```python
from build123d import *

# Parameters (mm, degrees)
SKETCH1_R                = 2
EXTRUDE1_DEPTH           = 3.125
ESBO_O1_R                = 12
ESBO_O1_R_2              = 2
RESSALTO_EXTRUS_O1_DEPTH = 1
FILETE1_R                = 1


with BuildPart() as part:
    # Sketch1 → Extrude1 (new body)
    with BuildSketch(Plane(origin=(0, 0, 0), x_dir=(1, 0, 0), z_dir=(0, 1, 0))):
        Polygon((3.859462612, 2.263930582), (-0.030890091, 4.474357958), (-3.890352703, 2.210427376), (-3.859462612, -2.263930582), (0.030890091, -4.474357958), (3.890352703, -2.210427376), align=None)
        with Locations(Location((0, 0, 0), (0, 0, 270))):  # turned: the seam where the file's is
            Circle(SKETCH1_R, mode=Mode.SUBTRACT)
    extrude(amount=EXTRUDE1_DEPTH)

    # Esboço1 → Ressalto-extrusão1 (add)
    with BuildSketch(Plane(origin=(0, 3.125, 0), x_dir=(1, 0, 0), z_dir=(0, 1, 0))):
        with Locations(Location((0, 0, 0), (0, 0, 270))):  # turned: the seam where the file's is
            Circle(ESBO_O1_R)
        with Locations(Location((0, 0, 0), (0, 0, 270))):  # turned: the seam where the file's is
            Circle(ESBO_O1_R_2, mode=Mode.SUBTRACT)
    extrude(amount=RESSALTO_EXTRUS_O1_DEPTH)

    # Filete1
    filete1_edges = [part.edges().sort_by_distance(p)[0] for p in [
        (-1.960621397, 3.125, -3.342392667),
        (-3.874907657, 3.125, 0.026751603),
        (-1.91428626, 3.125, 3.36914427),
        (1.960621397, 3.125, 3.342392667),
        (3.874907657, 3.125, -0.026751603),
        (1.91428626, 3.125, -3.36914427),
    ]]
    fillet(filete1_edges, radius=FILETE1_R)


solid = part.part
```
Source: CAD feature listing. Evaluate the final solid. Frame: model axes, mm. A direction names the side the tool comes from. Round coordinates to 2 decimals unless told otherwise and drop trailing zeros. Loops run counter-clockwise (first coordinate to the right, second up) from the corner with the lowest first, then second, coordinate; pieces in that order, holes last.
1. Contact query for flat-ended pins moving along their axis: pin 1 (4 mm diameter, centred on x = 8, z = -5, fed in from -Y) (3 decimals); pin 2 (12 mm diameter, centred on x = 5, z = -1, fed in from -Y); pin 3 (1 mm diameter, centred on y = 0.5, z = -0.5, fed in from +X). Output: stop coordinate, or through.
2. Section query D-D on z = 9.5. Output: boundary loops of the cut face in (x, y) (3 decimals).
3. Access query for faces 5 (the cylindrical face through (-4.16, 2.824, 0.068)), 6 (the cylindrical face through (4.16, 2.824, -0.068)), 7 (the flat face through (-1.93, 1.05, -3.36)). Directions: +Z, -Z, +X, -X, +Y, -Y. A direction counts if a zero-diameter tool reaches every point of the face in a straight line with its end or side. Return the directions, or none.
4. Section query B-B on x = -8.25. Output: boundary loops of the cut face in (y, z) (3 decimals), and give its area (3 significant figures).
5. Mould query, pull axis Z, two halves, no side actions, for faces 1 (the cylindrical face through (-2.021, 2.824, 3.637)), 2 (the flat face through (-5.2, 3.125, -0.2)), 3 (the cylindrical face through (3.604, 3.618, 11.446)), 4 (the cylindrical face through (-2, 2, 0)). Classes: released by +Z, released by -Z, zero draft, split by the parting line, or undercut.
6. Section query A-A on y = 1.1. Output: boundary loops of the cut face in (x, z), and give its area (3 significant figures).
7. Section query C-C on y = 2.65. Output: boundary loops of the cut face in (x, z).
8. Ray query, L1, parallel to X at y = 3.3, z = 0; L2, parallel to Y at x = 2.5, z = -10.5 (3 decimals); L3, parallel to X at y = 1.3, z = 0. Return the intervals inside material, ascending.
Answers below:
1. pin 1: stops at y = 3.125
1. pin 2: stops at y = 0
1. pin 3: stops at x = 3.88
2. outline: (-7.331, 3.125) - (7.331, 3.125) - (7.331, 4.125) - (-7.331, 4.125) - close
3. face 5: +Z, -X, -Y
3. face 6: -Z, +X, -Y
3. face 7: -Z, -X, -Y
4. outline: (3.125, -8.714) - (4.125, -8.714) - (4.125, 8.714) - (3.125, 8.714) - close
4. area: 17.4 mm2
5. face 1: released by +Z
5. face 2: zero draft
5. face 3: split by the parting line
5. face 4: undercut
6. outline: (-3.89, -2.21) - (-0.03, -4.47) - (3.86, -2.26) - (3.89, 2.21) - (0.03, 4.47) - (-3.86, 2.26) - close; hole circle Ø4 at (0, 0)
6. area: 39.4 mm2
7. outline: (-4.04, -2.3) - (-0.03, -4.65) - (4.01, -2.35) - (4.04, 2.3) - (0.03, 4.65) - (-4.01, 2.35) - close; hole circle Ø4 at (0, 0)
8. L1: x = -12 to -2, 2 to 12
8. L2: y = 3.125 to 4.125
8. L3: x = -3.88 to -2, 2 to 3.88
